Design review of the part built by this model. Coordinates are the model's own, in mm. A direction names the side the tool comes from. Give positions to 0.01 mm unless a question says otherwise; leave off trailing zeros. Loops run counter-clockwise (first coordinate to the right, second up) from the corner with the lowest first, then second, coordinate; pieces in that order, holes last. Notation, with made-up numbers: (-18.5, 5.5) -> (24.5, 5.5) arc R15 ccw to (24.5, 30.5) -> close; hole circle Ø10 at (-31, 1). An arc over 180 degrees is marked (long way). Answer as CSV lines item,"result".
from build123d import *

# Parameters (mm, degrees)
SKETCH1_R           = 17
BOSS_EXTRUDE1_DEPTH = 20
SKETCH2_R           = 16
CUT_EXTRUDE1_DEPTH  = 3
SKETCH3_R           = 1
CUT_EXTRUDE2_DEPTH  = 2
FILLET1_R           = 1


with BuildPart() as part:
    # Sketch1 → Boss-Extrude1 (new body)
    with BuildSketch(Plane(origin=(0, 0, 0), x_dir=(1, 0, 0), z_dir=(0, 1, 0))):
        Circle(SKETCH1_R)
    extrude(amount=BOSS_EXTRUDE1_DEPTH)

    # Sketch2 → Cut-Extrude1 (cut)
    with BuildSketch(Plane(origin=(0, 20, 0), x_dir=(1, 0, 0), z_dir=(0, 1, 0))):
        Circle(SKETCH2_R)
    extrude(amount=-CUT_EXTRUDE1_DEPTH, mode=Mode.SUBTRACT)

    # Sketch3 → Cut-Extrude2 (cut)
    with BuildSketch(Plane.XZ):
        Circle(SKETCH3_R)
    extrude(amount=-CUT_EXTRUDE2_DEPTH, mode=Mode.SUBTRACT)

    # Fillet1
    fillet1_edges = [part.edges().sort_by_distance(p)[0] for p in [
        (-1, 2, 0),
    ]]
    fillet(fillet1_edges, radius=FILLET1_R)


solid = part.part
Q1. For faces 1 (the flat face through (4, 0, 0)), 2 (the flat face through (0, 17, 0)), list the 3-axis set-ups (+Z, -Z, +X, -X, +Y, -Y) from which the entire face can be reached by the end or side of a thin tool; tool diameter is ignored.
Filled sheet:
face 1,"+Z, -Z, +X, -X, -Y"
face 2,"+Y"
Q2. Clearance check with flat-ended pins moving along their axes: pin 1 Ø1.5 at (y, z) = (11, -13) entering from -X; pin 2 Ø1.5 at (y, z) = (10, -10) entering from -X; pin 3 Ø3 at (x, y) = (-8.5, 14.5) entering from -Z. State where each tip first meets the part, or that it passes through.
Filled sheet:
pin 1,"stops at x = -11.79"
pin 2,"stops at x = -14.26"
pin 3,"stops at z = -15.49"
Q3. To check wall thickness, follow probe 1 along Z at (x, y) = (0, 0.2); probe 2 along Z at (x, y) = (0, 18.45). State the ranges of each line that lie inside material, in increasing order. Write a range as from..to.
Filled sheet:
probe 1,"z = -17..-1, 1..17"
probe 2,"z = -17..-16, 16..17"
Q4. We need section C-C, the plane y = 3.25. State the section outline as (x, z) points.
Filled sheet:
outline,"circle Ø34 at (0, 0)"
Q5. We need section B-B, the plane z = 0. State the section outline as (x, y) points.
Filled sheet:
outline,"(-17, 0) -> (-1, 0) -> (-1, 1) arc R1 cw to (1, 1) -> (1, 0) -> (17, 0) -> (17, 20) -> (16, 20) -> (16, 17) -> (-16, 17) -> (-16, 20) -> (-17, 20) -> close"
Q6. The part is to be moulded in two halves that separate along Z. For faces 3 (the cylindrical face through (9.139, 9.86, -14.334)), 4 (the flat face through (13, 20, 10)), 5 (the cylindrical face through (-0.217, 0.493, -0.976)), say which applies: pulls with the +Z half, pulls with the -Z half, needs draft (parallel to the pull), parting line crosses it, or undercut.
Filled sheet:
face 3,"parting line crosses it"
face 4,"needs draft"
face 5,"undercut"
Q7. We need section A-A, the plane x = 0. State the section outline as (y, z) points.
Filled sheet:
outline,"(0, -17) -> (20, -17) -> (20, -16) -> (17, -16) -> (17, 16) -> (20, 16) -> (20, 17) -> (0, 17) -> (0, 1) -> (1, 1) arc R1 cw to (1, -1) -> (0, -1) -> close"
Q8. We need section D-D, the plane x = 5.5. State the section outline as (y, z) points, and give its area (3 significant figures).
Filled sheet:
outline,"(0, -16.09) -> (20, -16.09) -> (20, -15.02) -> (17, -15.02) -> (17, 15.02) -> (20, 15.02) -> (20, 16.09) -> (0, 16.09) -> close"
area,"553 mm^2"
